```python
from build123d import *

# Parameters (mm, degrees)
F0_R     = 5
F0_R_2   = 4.4774041187
F1_DEPTH = 15


with BuildPart() as f1:
    # F0 (on Front) → F1 (new body)
    with BuildSketch(Plane.XZ):
        with BuildLine():
            Line((49.9977292464, 9.523481164), (0.1905988779, 9.9981834384))
            ThreePointArc((0.1905988779, 9.9981834384), (7.1381366189, 7.0033567388), (10, 0))
            ThreePointArc((10, 0), (7.1381366189, -7.0033567388), (0.1905988779, -9.9981834384))
            Line((0.1905988779, -9.9981834384), (49.9977292464, -9.523481164))
            ThreePointArc((49.9977292464, -9.523481164), (40.3830490678, 0), (49.9977292464, 9.523481164))
        make_face()
        with BuildLine():
            Line((0.1905988779, 9.9981834384), (0, 10))
            ThreePointArc((0, 10), (-10, 0), (0, -10))
            Line((0, -10), (0.1905988779, -9.9981834384))
            ThreePointArc((0.1905988779, -9.9981834384), (7.1381366189, -7.0033567388), (10, 0))
            ThreePointArc((10, 0), (7.1381366189, 7.0033567388), (0.1905988779, 9.9981834384))
        make_face()
        Circle(F0_R, mode=Mode.SUBTRACT)
        with BuildLine():
            ThreePointArc((59.4308764543, 0), (56.6734014185, 6.7022563314), (49.9977292464, 9.523481164))
            ThreePointArc((49.9977292464, 9.523481164), (40.3830490678, 0), (49.9977292464, -9.523481164))
            ThreePointArc((49.9977292464, -9.523481164), (56.6734014185, -6.7022563314), (59.4308764543, 0))
        make_face()
        with Locations((49.9069627611, 0)):
            Circle(F0_R_2, mode=Mode.SUBTRACT)
    extrude(amount=F1_DEPTH)


solid = f1.part
```
Geometry: final body of the model. Coordinates: model frame, mm. Give positions to 0.01 mm unless a question says otherwise; leave off trailing zeros. Order: outer loops, then holes, each group sorted by start corner. A loop starts at its lowest first (then second) coordinate and runs counter-clockwise, first axis right, second up. Notation, with made-up numbers: (35, -10) -> (83, -10) arc R9 ccw to (83, 3) -> close; hole circle Ø8 at (59, -23). An arc over 180 degrees is marked (long way). Write each question's results on one line, items separated by ' | '. Start each with the question number.
1) Line query: line 1 (X direction, y = -13, z = 0.25); line 2 (Z direction, x = 0, y = -8.5); line 3 (X direction, y = -11.5, z = 1.25). Output: solid intervals per line, ascending. Write a range as from..to.
2) Section A-A (y = -7.25). Return loops of the section in (x, z).
3) Draft query along Z for faces 1 (the cylindrical face through (54.043, -7.395, -1.715)), 2 (the cylindrical face through (-10, -7, 0)), 3 (the flat face through (24, -15, 0)), 4 (the cylindrical face through (-1.08, -7.4, -4.88)). Return one class per face: pulls with the +Z half, pulls with the -Z half, needs draft (parallel to the pull), parting line crosses it, or undercut.
4) Section C-C (x = 46.5). Return loops of the section in (y, z).
5) Section D-D (x = 32.5). Return loops of the section in (y, z), then the cut area to 3 significant figures.
6) Section B-B (x = 2). Return loops of the section in (y, z).
7) First-contact query: pin 1 (2 mm diameter, centred on x = 22, y = -5.5, fed in from +Z); pin 2 (4 mm diameter, centred on y = -3.5, z = -5.5, fed in from +X); pin 3 (2 mm diameter, centred on y = -5.5, z = -5.5, fed in from +X). Flat tips, straight axial feed; report the tip coordinate or a pass-through.
Calculated:
1) line 1: -10..-4.99, 4.99..45.44, 54.38..59.43 | line 2: -10..-5, 5..10 | line 3: -9.92..-4.84, 4.84..45.61, 54.21..59.35
2) outline: (0, -10) -> (50, -9.52) arc R9.52 ccw to (50, 9.52) -> (0, 10) arc R10 ccw to start; hole circle Ø10 at (0, 0); hole circle Ø8.95 at (49.91, 0)
3) face 1: undercut | face 2: parting line crosses it | face 3: needs draft | face 4: undercut
4) outline: (-15, -9.56) -> (0, -9.56) -> (0, -2.91) -> (-15, -2.91) -> close; (-15, 2.91) -> (0, 2.91) -> (0, 9.56) -> (-15, 9.56) -> close
5) outline: (-15, -9.69) -> (0, -9.69) -> (0, 9.69) -> (-15, 9.69) -> close | area: 291 mm2
6) outline: (-15, -9.98) -> (0, -9.98) -> (0, -4.58) -> (-15, -4.58) -> close; (-15, 4.58) -> (0, 4.58) -> (0, 9.98) -> (-15, 9.98) -> close
7) pin 1: z = 9.8 | pin 2: x = 58.76 | pin 3: x = 58.3
